Verification items for this drawing (mm, ordinates from the low corner). Coordinates: 2 decimals unless noted, no trailing zeros. Write each loop counter-clockwise with the first axis right and the second up, starting at its lowest first coordinate (ties: lowest second). Pieces come first, ordered by that corner, then holes. Notation, with made-up numbers: (53, 34.25) -> (111, 34.25) arc R30 cw to (111, 70.25) -> close; hole circle Ø2 at (76, 76.25). An arc over 180 degrees is marked (long way). Answer as CSV lines item,"result".
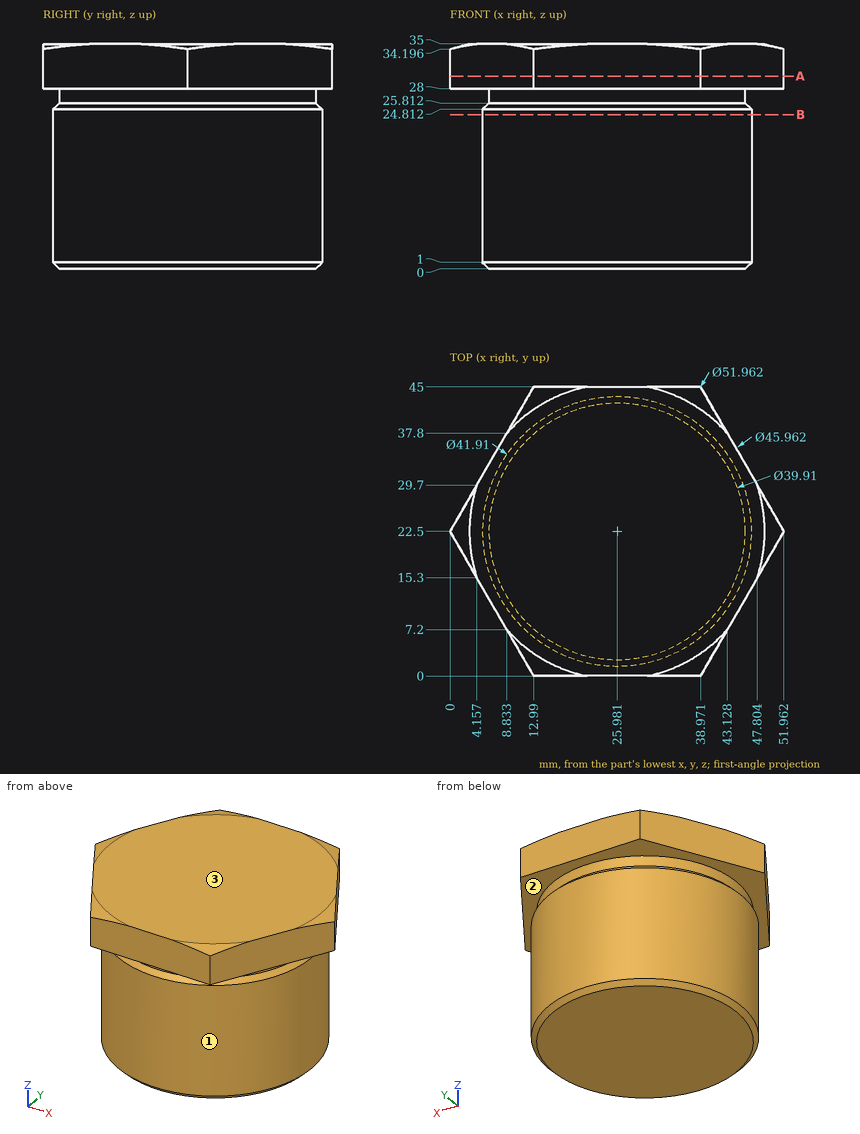
Item 1: Depth check by flat-ended pin: pin 1 Ø1 at (y, z) = (32, 18.5) entering from -X; pin 2 Ø8 at (x, z) = (43.5, 10) entering from -Y; pin 3 Ø5 at (y, z) = (24.5, 9) entering from +X. Enter the tip coordinate at first touch or a pass-through.
Responses:
pin 1,"stops at x = 7.06"
pin 2,"stops at y = 6.49"
pin 3,"stops at x = 46.94"
Item 2: Thickness scan on probe 1 along X at (y, z) = (23, 10); probe 2 along Y at (x, z) = (26, 19) (1 decimal); probe 3 along X at (y, z) = (36, 33) (1 decimal). Record the ranges inside material, lowest first.
Responses:
probe 1,"x = 5.03 to 46.93"
probe 2,"y = 1.5 to 43.5"
probe 3,"x = 7.8 to 44.2"
Item 3: Cross-section at A-A, the plane z = 30. Record the cut outline in (x, y), plus the area to 3 significant figures.
Responses:
outline,"(0, 22.5) -> (12.99, 0) -> (38.97, 0) -> (51.96, 22.5) -> (38.97, 45) -> (12.99, 45) -> close"
area,"1,750 mm2"
Item 4: Cross-section at B-B, the plane z = 24. Record the cut outline in (x, y) (1 decimal).
Responses:
outline,"circle Ø41.9 at (26, 22.5)"
Item 5: Release check for a two-part mould opening along Z. For the marked faces 1, 2 and 3 record: +Z half, -Z half, draft (parallel to the pull), parting line (faces both ways), or undercut.
Responses:
face 1,"draft"
face 2,"undercut"
face 3,"+Z half"
